CAD build for the part. Positions are in the model's coordinates, mm. Face numbers are marked on the shaded views. Give positions to 0.01 mm unless a question says otherwise; leave off trailing zeros. Write each loop counter-clockwise with the first axis right and the second up, starting at its lowest first coordinate (ties: lowest second). Pieces come first, ordered by that corner, then holes. Notation, with made-up numbers: (-7.75, -33) -> (8.25, -33) arc R12 cw to (8.25, -18) -> close; hole circle Ø2 at (59, 86). An arc over 180 degrees is marked (long way). Answer as a JSON object with one key per item and string values.
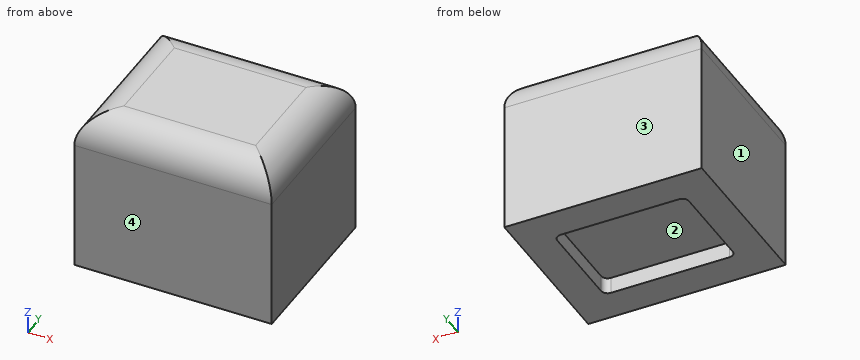
```python
from build123d import *

# Parameters (mm, degrees)
F0_W     = 60
F0_H     = 50
F1_DEPTH = 50
F2_W     = 40
F2_H     = 30
F3_DEPTH = 5
F4_R     = 2
F5_R     = 10


with BuildPart() as f1:
    # F0 (on Top) → F1 (new body)
    with BuildSketch(Plane.XY):
        with Locations((30, 25)):
            Rectangle(F0_W, F0_H)
    extrude(amount=F1_DEPTH)

    # F2 (on face) → F3 (cut)
    with BuildSketch(Plane(origin=(0, 0, 0), x_dir=(1, 0, 0), z_dir=(0, 0, -1))):
        with Locations((30, -25)):
            Rectangle(F2_W, F2_H)
    extrude(amount=-F3_DEPTH, mode=Mode.SUBTRACT)

    # F4
    f4_edges = [f1.edges().sort_by_distance(p)[0] for p in [
        (50, 40, 2.5),
        (10, 40, 2.5),
        (10, 10, 2.5),
        (50, 10, 2.5),
    ]]
    fillet(f4_edges, radius=F4_R)

    # F5
    f5_edges = [f1.edges().sort_by_distance(p)[0] for p in [
        (0, 25, 50),
        (30, 0, 50),
        (60, 25, 50),
        (30, 50, 50),
    ]]
    fillet(f5_edges, radius=F5_R)


solid = f1.part
```
1) Mould opens along Y. For the marked faces 1, 2, 3 and 4 say: released by +Y, released by -Y, zero draft, split by the parting line, or undercut.
Model answer:
{"face 1": "zero draft", "face 2": "undercut", "face 3": "released by +Y", "face 4": "released by -Y"}
2) Pin check, flat tips, straight feed: pin 1 (1 mm diameter, centred on x = 47, y = 39, fed in from -Z); pin 2 (5 mm diameter, centred on x = 48.5, y = 6.5, fed in from +Z). Stop position of each tip, or through.
Model answer:
{"pin 1": "stops at z = 5", "pin 2": "stops at z = 49.95"}
3) Slice it at A-A (z = 4). List the corners of the cut face in (x, y), then the cut area to 3 significant figures.
Model answer:
{"outline": "(0, 0) -> (60, 0) -> (60, 50) -> (0, 50) -> close; hole (10, 12) arc R2 ccw to (12, 10) -> (48, 10) arc R2 ccw to (50, 12) -> (50, 38) arc R2 ccw to (48, 40) -> (12, 40) arc R2 ccw to (10, 38) -> close", "area": "1,800 mm2"}
4) Slice it at B-B (x = 40.5). List the corners of the cut face in (y, z).
Model answer:
{"outline": "(0, 0) -> (10, 0) -> (10, 5) -> (40, 5) -> (40, 0) -> (50, 0) -> (50, 40) arc R10 ccw to (40, 50) -> (10, 50) arc R10 ccw to (0, 40) -> close"}
5) Wall check: probe 1 along X at (y, z) = (21.5, 4); probe 2 along Z at (x, y) = (19.5, 15); probe 3 along Y at (x, z) = (46, 45). Give the ranges that are in metal, low to high.
Model answer:
{"probe 1": "x = 0 to 10, 50 to 60", "probe 2": "z = 5 to 50", "probe 3": "y = 1.34 to 48.66"}
6) Slice it at D-D (z = 46). List the corners of the cut face in (x, y), then the cut area to 3 significant figures.
Model answer:
{"outline": "(2, 2) -> (58, 2) -> (58, 48) -> (2, 48) -> close", "area": "2,580 mm2"}
7) Slice it at C-C (y = 39). List the corners of the cut face in (x, z).
Model answer:
{"outline": "(0, 0) -> (10.27, 0) -> (10.27, 5) -> (49.73, 5) -> (49.73, 0) -> (60, 0) -> (60, 40) arc R10 ccw to (50, 50) -> (10, 50) arc R10 ccw to (0, 40) -> close"}
